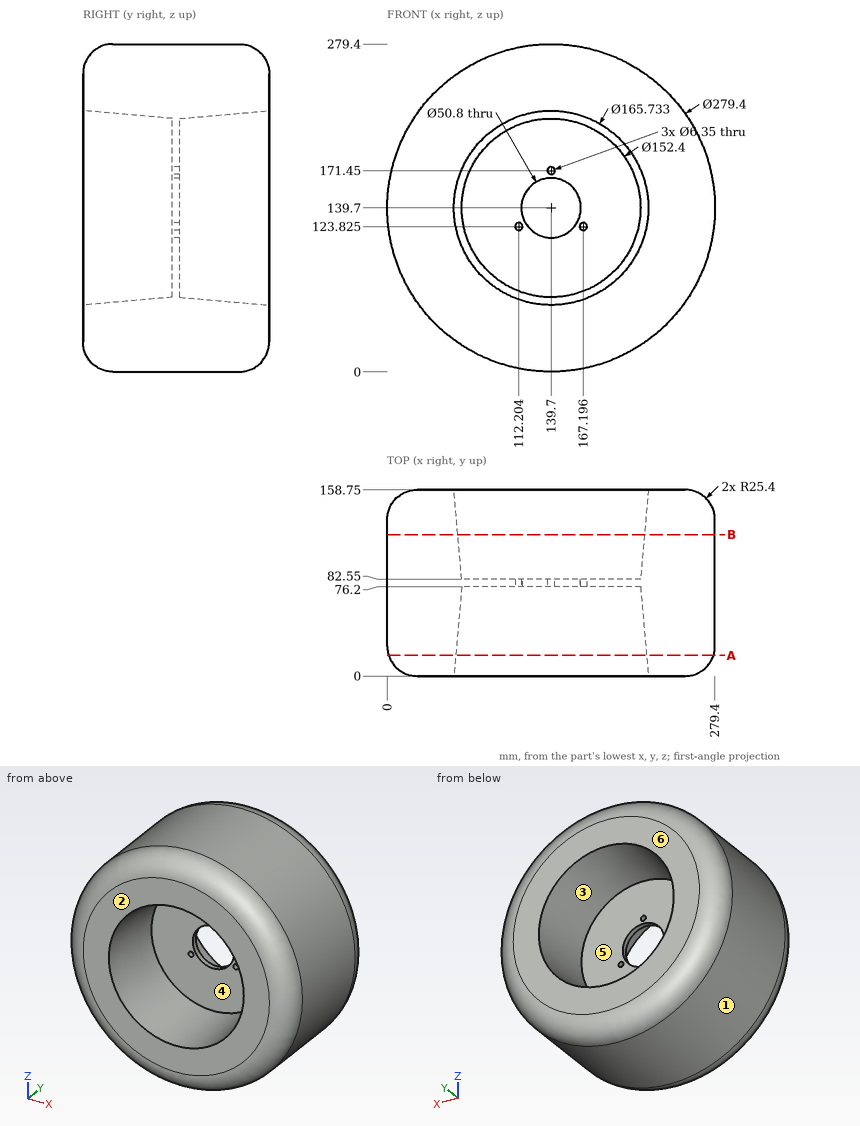
Geometry check sheet. Reference: drawing and pictorial views, mm from the part's lowest x, y, z. A direction names the side the tool comes from. Give positions to 0.01 mm unless a question says otherwise; leave off trailing zeros. Write each loop counter-clockwise with the first axis right and the second up, starting at its lowest first coordinate (ties: lowest second). Pieces come first, ordered by that corner, then holes. Notation, with made-up numbers: M -4,64.25 L 39,64.25 A32 cw 39,101.25 Z; hole C -19,29 d11. An arc over 180 degrees is marked long. Answer as CSV lines item,"result". Start each with the question number.
Q1. Tool access check on the marked faces 4, 5 and 6. Record the directions out of +Z, -Z, +X, -X, +Y, -Y that give a thin tool (end or side, any length) a straight path to the whole face; none if there is none.
Q2. Section check A-A, the plane y = 17.5. Record the cut outline in (x, z) (1 decimal), then the cut area to 3 significant figures.
Q3. Go/stop test with flat-tipped pins: pin 1 (8 mm diameter, centred on x = 78, z = 164.5, fed in from -Y); pin 2 (12 mm diameter, centred on x = 114.5, y = 68.5, fed in from +Z); pin 3 (10 mm diameter, centred on y = 124.5, z = 235.5, fed in from -X). Record where each tip stops, or that it passes through.
Q4. Release check for a two-part mould opening along Z. For the marked faces 1, 2 and 3 record: pulls with the +Z half, pulls with the -Z half, needs draft (parallel to the pull), parting line crosses it, or undercut.
Q5. Material ranges on L1, parallel to Z at x = 139.7, y = 78.5 (1 decimal); L2, parallel to Z at x = 139, y = 80; L3, parallel to Z at x = 94, y = 84 (1 decimal), recorded low to high.
Q6. Section check B-B, the plane y = 120.5. Record the cut outline in (x, z).
Geometry says:
1,face 4,"-Y"
1,face 5,"+Y"
1,face 6,"+Z, -Z, +X, -X, +Y"
2,outline,"C 139.7,139.7 d276.9; hole C 139.7,139.7 d162.7"
2,area,"39,400 mm^2"
3,pin 1,"y = 76.2"
3,pin 2,"z = 278.07"
3,pin 3,"x = 33.53"
4,face 1,"parting line crosses it"
4,face 2,"needs draft"
4,face 3,"undercut"
5,L1,"0 to 114.3, 165.1 to 168.3, 174.6 to 279.4"
5,L2,"0 to 114.31, 165.09 to 168.35, 174.55 to 279.4"
5,L3,"7.7 to 78.6, 200.8 to 271.7"
6,outline,"C 139.7,139.7 d279.4; hole C 139.7,139.7 d159.04"
